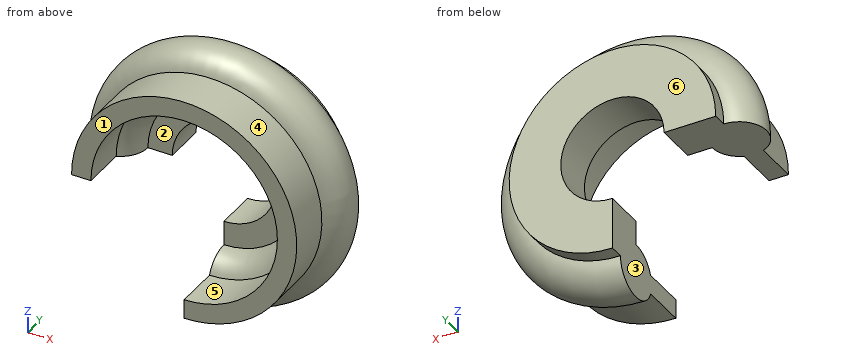
Autodesk Inventor part; units mm, degrees
ref_plane "YZ Plane" through (0, 0, 0) normal (1, 0, 0) x (0, 1, 0)
ref_plane "XZ Plane" through (0, 0, 0) normal (0, 1, 0) x (-1, 0, 0)
ref_plane "XY Plane" through (0, 0, 0) normal (0, 0, 1) x (1, 0, 0)
sketch "Sketch1" plane through (0, 0, 0) normal (1, 0, 0) x (0, 1, 0)
  line L0 (21.8125, -13.0228) -> (14.2915, -13.0228)
  line L1 (14.2915, -13.0228) -> (14.2915, -22.4132)
  line L2 (14.2915, -22.4132) -> (21.8125, -22.4132)
  line L3 (21.8125, -22.4132) -> (21.8125, -13.0228)
  circle A0 centre (14.2915, -22.4132) radius 4.9585
  line L4 (11.1179, -20.5873) -> (1.6405, -20.5873)
  line L5 (1.6405, -20.5873) -> (1.6405, -24.1087)
  line L6 (1.6405, -24.1087) -> (11.1179, -24.1087)
  line L7 (11.1179, -24.1087) -> (11.1179, -20.5873)
  line L8 (21.8125, -3.6323) -> (0.6841, -3.6323)
  point P0 (0, 0)
  point P1 (14.2915, -17.4546)
  point P2 (9.6814, -20.5873)
  point P3 (9.6319, -24.1087)
  point P4 (19.25, -22.4132)
revolve "Revolution1" add sketch "Sketch1" angle 270 about axis through (0, 21.8125, -3.6323) along (0, -1, 0)
properties part number "odd revolve"
Geometry: final body of the model. Coordinates: model frame, mm. Face numbers are marked on the shaded views. A direction names the side the tool comes from. Round coordinates to 2 decimals unless told otherwise and drop trailing zeros. Order: outer loops, then holes, each group sorted by start corner. A loop starts at its lowest first (then second) coordinate and runs counter-clockwise, first axis right, second up. Notation, with made-up numbers: M 31,22.25 L 54,22.25 A23 cw 54,59.25 Z; hole C 75.25,-33 d4. An arc over 180 degrees is marked long. One line per item, written item: value.
(1) Line query: probe 1 along Z at (x, y) = (13.5, 4); probe 2 along X at (y, z) = (4.5, 0); probe 3 along Z at (x, y) = (11, 6.5). Output: solid intervals per line, ascending. Write a range as [from, to].
Result sheet:
probe 1: [-19.03, -13.89], [6.63, 11.76]
probe 2: [-20.15, -16.56], [16.56, 20.15]
probe 3: [-20.9, -16.53], [9.27, 13.64]
(2) Cut plane B-B (y = 16.25). Return the cut outline in (x, z).
Result sheet:
outline: M -23.34,-3.63 L -9.39,-3.63 A9.39 cw long 0,-13.02 L 0,-26.97 A23.34 ccw long Z
(3) Cut plane A-A (y = 7.5). Return the cut outline in (x, z) (3 decimals), and give its area (3 significant figures).
Result sheet:
outline: M -20.476,-3.632 L -16.955,-3.632 A16.955 cw long 0,-20.587 L 0,-24.109 A20.476 ccw long Z
area: 311 mm2
(4) Pin query (flat end, axial travel): P1, Ø1, axis at x = 13, z = -8, coming from the -Y side; P2, Ø1, axis at y = 16, z = -19.5, coming from the +X side; P3, Ø1, axis at x = -9.5, y = 15.5, coming from the +Z side; P4, Ø1, axis at x = 1, z = 3.5, coming from the -Y side. Return the tip coordinate at first contact, or that it passes through.
Result sheet:
P1: y = 12.36
P2: x = 17.75
P3: z = 18.21
P4: through
(5) Pull-direction query (X, two-part tool) for the marked faces 4, 5 and 6; classes: pulls with the +X half, pulls with the -X half, needs draft (parallel to the pull), parting line crosses it, or undercut.
Result sheet:
face 4: parting line crosses it
face 5: undercut
face 6: needs draft
(6) Reachability of the marked faces 1, 2 and 3 from +Z, -Z, +X, -X, +Y, -Y: full face, straight path, thin tool, end or side. Return the list, or none.
Result sheet:
face 1: +Z, -Z, +X, -X, -Y
face 2: -Y
face 3: -Z, -X, +Y, -Y
